from build123d import *

# Parameters (mm, degrees)
SKETCH2_W = 12.5
SKETCH2_H = 60
FILLET1_R = 0.3


with BuildPart() as part:
    # Sketch2 → Revolve1 (revolve)
    with BuildSketch(Plane.XY, mode=Mode.PRIVATE) as revolve1_sk:
        with Locations((6.25, 0)):
            Rectangle(SKETCH2_W, SKETCH2_H)
    revolve(revolve1_sk.sketch.rotate(Axis((0, 30, 0), (0, -1, 0)), 90), axis=Axis((0, 30, 0), (0, -1, 0)))

    # Sketch4 → Cut-Revolve1 (revolve, cut)
    with BuildSketch(Plane.XY, mode=Mode.PRIVATE) as cut_revolve1_sk:
        Polygon((0, 30), (0, 29), (1, 29.5), (1, 30), align=None)
    cut_revolve1 = revolve(cut_revolve1_sk.sketch.rotate(Axis((0, 30, 0), (0, -1, 0)), 180), axis=Axis((0, 30, 0), (0, -1, 0)), mode=Mode.SUBTRACT)

    # Mirror2: Cut-Revolve1 across plane
    add(cut_revolve1.mirror(Plane.ZX), mode=Mode.SUBTRACT)

    # Fillet1
    fillet1_edges = [part.edges().sort_by_distance(p)[0] for p in [
        (1, -30, 0),
        (0, -30, -12.5),
        (0, 30, -12.5),
        (1, 30, 0),
    ]]
    fillet(fillet1_edges, radius=FILLET1_R)


solid = part.part
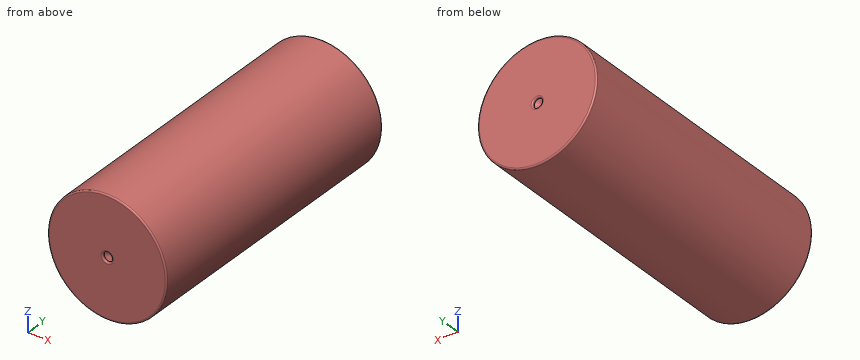
The listing builds one solid part. Answer for the finished solid, in the listing's coordinates (mm). Round coordinates to 2 decimals unless told otherwise and drop trailing zeros. Order: outer loops, then holes, each group sorted by start corner. A loop starts at its lowest first (then second) coordinate and runs counter-clockwise, first axis right, second up. Notation, with made-up numbers: M -32,45 L -23,45 A12 cw -23,53 Z; hole C 60.25,0.25 d11. An arc over 180 degrees is marked long. Answer in a Markdown table with one row per item. Add a question column.
1) Consider line 1 along X through (y, z) = (-3.5, 4.25); line 2 along X through (y, z) = (-15, 9.5); line 3 along Z through (x, y) = (0.75, 27.5). Determine where each line is inside the solid, lowest interval first. Write a range as from..to.
2) The part is cut by section A-A on y = 9.5. Determine the outline of the cut face in (x, z), plus the area to 3 significant figures.
3) Flat-ended cylindrical pins translate along their axes: pin 1 Ø3 at (x, y) = (10, -2.5) entering from -Z; pin 2 Ø3 at (y, z) = (-12, 7.5) entering from -X; pin 3 Ø1.2 at (x, z) = (0, 0) entering from -Y. Find the tip coordinate at first contact, or state that the pin passes through.
Findings below:
| question | item | result |
|---|---|---|
| 1 | line 1 | x = -11.76..11.76 |
| 1 | line 2 | x = -8.12..8.12 |
| 1 | line 3 | z = -12.48..12.48 |
| 2 | outline | C 0,0 d25 |
| 2 | area | 491 mm² |
| 3 | pin 1 | stops at z = -9.17 |
| 3 | pin 2 | stops at x = -10.97 |
| 3 | pin 3 | stops at y = -29.3 |
